from build123d import *

# Parameters (mm, degrees)
SKETCH1_R               = 1.35
BOSS_EXTRUDE1_DEPTH     = 21.5
SKETCH2_R               = 1.4
CUT_EXTRUDE1_DEPTH      = 21.5
SKETCH3_W               = 10.5
SKETCH3_H               = 10.75
CUT_EXTRUDE2_DEPTH      = 2
CUT_EXTRUDE2_DEPTH_BACK = 6


with BuildPart() as part:
    # Sketch1 → Boss-Extrude1 (new body)
    with BuildSketch(Plane(origin=(0, 0, 0), x_dir=(1, 0, 0), z_dir=(0, 1, 0))):
        Polygon((42.5, -2.5), (-42.5, -2.5), (-42.5, 2.5), (-32, 2.5), (-32, 3.5), (-17, 3.5), (-17, 2.5), (17, 2.5), (17, 3.5), (32, 3.5), (32, 2.5), (42.5, 2.5), align=None)
        with Locations((-39.5, 0)):
            Circle(SKETCH1_R, mode=Mode.SUBTRACT)
        with Locations((39.5, 0)):
            Circle(SKETCH1_R, mode=Mode.SUBTRACT)
    extrude(amount=BOSS_EXTRUDE1_DEPTH)

    # Sketch2 → Cut-Extrude1 (cut)
    with BuildSketch(Plane(origin=(0, 0, 2.5), x_dir=(-1, 0, 0), z_dir=(0, 0, -1))):
        with Locations((-7.5, 3)):
            Circle(SKETCH2_R)
        with Locations((7.5, 3)):
            Circle(SKETCH2_R)
        with Locations((-25, 3)):
            Circle(SKETCH2_R)
        with Locations((25, 3)):
            Circle(SKETCH2_R)
    extrude(amount=CUT_EXTRUDE1_DEPTH, mode=Mode.SUBTRACT)

    # Sketch3 → Cut-Extrude2 (cut, two sides)
    with BuildSketch(Plane(origin=(0, 0, -2.5), x_dir=(-1, 0, 0), z_dir=(0, 0, -1))) as cut_extrude2_sk:
        with Locations((-37.25, 5.375)):
            Rectangle(SKETCH3_W, SKETCH3_H)
        with Locations((37.25, 5.375)):
            Rectangle(SKETCH3_W, SKETCH3_H)
    extrude(amount=CUT_EXTRUDE2_DEPTH, mode=Mode.SUBTRACT)
    extrude(cut_extrude2_sk.sketch, amount=-CUT_EXTRUDE2_DEPTH_BACK, mode=Mode.SUBTRACT)


solid = part.part
The listing builds one solid part. Answer for the finished solid, in the listing's coordinates (mm). A direction names the side the tool comes from. Give positions to 0.01 mm unless a question says otherwise; leave off trailing zeros. Write each loop counter-clockwise with the first axis right and the second up, starting at its lowest first coordinate (ties: lowest second). Pieces come first, ordered by that corner, then holes.
1) Section C-C (x = -25) is taken. Write down the section's boundary in (y, z).
2) Section B-B (y = 17) is taken. Write down the section's boundary in (x, z).
3) Section D-D (y = 3) is taken. Write down the section's boundary in (x, z).
4) For a pull along X with two mould halves and no side action, classify faces 5 (the face through (-42.5, 16, 0)), 6 (the face through (0, 11, -2.5)), 7 (the face through (37, 10.75, 0)) as pulls with the +X half, pulls with the -X half, needs draft (parallel to the pull), parting line crosses it, or undercut.
5) A tool of negligible diameter and unlimited length cuts with its end or side. For faces 1 (the face through (-37, 10.75, 0)), 2 (the face through (37, 16, -2.5)), 3 (the face through (-25, 11, -3.5)), 4 (the face through (-37, 16, -2.5)), from which of +Z, -Z, +X, -X, +Y, -Y can it reach the whole face along a straight path? Write none if from no direction.
6) Section A-A (z = 0) is taken. Write down the section's boundary in (x, y), and give its area (3 significant figures).
7) Find the intervals of material crossed by L1, parallel to X at y = 3, z = -1.9; L2, parallel to X at y = 17.25, z = 0; L3, parallel to Z at x = -39.5, y = 13, in increasing order.
8) Given P1, Ø11.5, axis at x = -35.5, y = 14.5, coming from the -Z side; P2, Ø3, axis at y = 5.5, z = 0.5, coming from the +X side; P3, Ø6, axis at x = 4, y = 8, coming from the -Z side; P4, Ø3, axis at x = 39.5, z = 0, coming from the -Y side, each flat-ended and moving along its own axis, determine where each tip first touches the part or whether it passes through.
Response:
1. outline: (0, -3.5) - (1.6, -3.5) - (1.6, 2.5) - (0, 2.5) - close; (4.4, -3.5) - (21.5, -3.5) - (21.5, 2.5) - (4.4, 2.5) - close
2. outline: (-42.5, -2.5) - (-32, -2.5) - (-32, -3.5) - (-17, -3.5) - (-17, -2.5) - (17, -2.5) - (17, -3.5) - (32, -3.5) - (32, -2.5) - (42.5, -2.5) - (42.5, 2.5) - (-42.5, 2.5) - close; hole circle Ø2.7 at (-39.5, 0); hole circle Ø2.7 at (39.5, 0)
3. outline: (-32, -3.5) - (-26.4, -3.5) - (-26.4, 2.5) - (-32, 2.5) - close; (-23.6, -3.5) - (-17, -3.5) - (-17, -2.5) - (-8.9, -2.5) - (-8.9, 2.5) - (-23.6, 2.5) - close; (-6.1, -2.5) - (6.1, -2.5) - (6.1, 2.5) - (-6.1, 2.5) - close; (8.9, -2.5) - (17, -2.5) - (17, -3.5) - (23.6, -3.5) - (23.6, 2.5) - (8.9, 2.5) - close; (26.4, -3.5) - (32, -3.5) - (32, 2.5) - (26.4, 2.5) - close
4. face 5: pulls with the -X half
4. face 6: undercut
4. face 7: needs draft
5. face 1: +Z, -Z, -X, -Y
5. face 2: -Z, +X, +Y, -Y
5. face 3: -Z, +X, -X, +Y, -Y
5. face 4: -Z, -X, +Y, -Y
6. outline: (-42.5, 10.75) - (-40.85, 10.75) - (-40.85, 21.5) - (-42.5, 21.5) - close; (-38.15, 10.75) - (-32, 10.75) - (-32, 0) - (32, 0) - (32, 10.75) - (38.15, 10.75) - (38.15, 21.5) - (-38.15, 21.5) - close; (40.85, 10.75) - (42.5, 10.75) - (42.5, 21.5) - (40.85, 21.5) - close; hole circle Ø2.8 at (-25, 3); hole circle Ø2.8 at (-7.5, 3); hole circle Ø2.8 at (7.5, 3); hole circle Ø2.8 at (25, 3)
6. area: 1,520 mm2
7. L1: x = -32 to -26.4, -23.6 to -8.9, -6.1 to 6.1, 8.9 to 23.6, 26.4 to 32
7. L2: x = -42.5 to -40.85, -38.15 to 38.15, 40.85 to 42.5
7. L3: z = -2.5 to -1.35, 1.35 to 2.5
8. P1: stops at z = -3.5
8. P2: stops at x = 32
8. P3: stops at z = -2.5
8. P4: stops at y = 10.75
